Check sheet for the drawn part. Datum: minimum x, y, z corner. Units: mm. Round coordinates to 2 decimals unless told otherwise and drop trailing zeros. Loops run counter-clockwise (first coordinate to the right, second up) from the corner with the lowest first, then second, coordinate; pieces in that order, holes last. Notation, with made-up numbers: (-13.5, 25) -> (35.5, 25) arc R22 ccw to (35.5, 46) -> close; hole circle Ø7 at (-3.75, 18). An arc over 180 degrees is marked (long way). Write item = value, one per line. Start each with the question number.
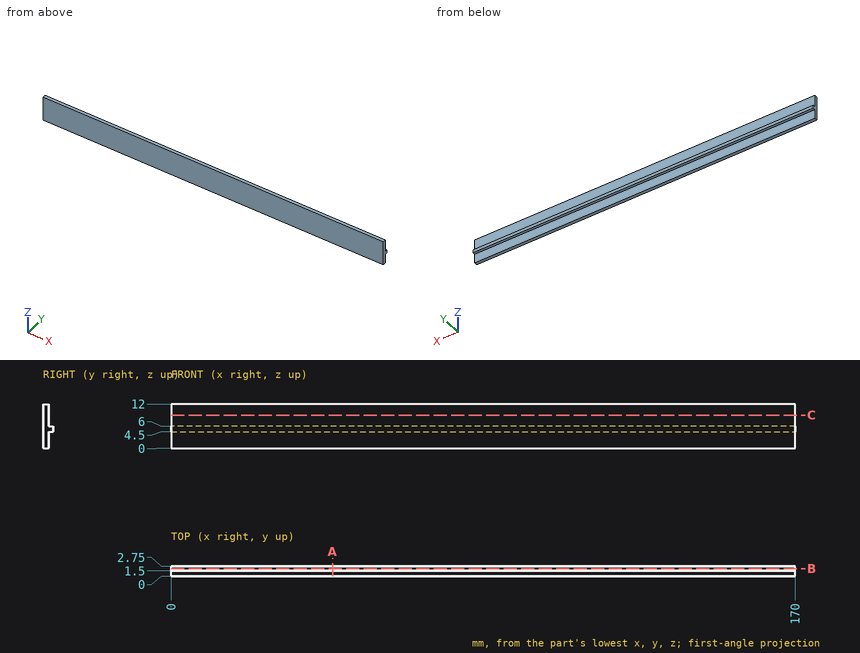
(1) Scan lines: line 1 (Y direction, x = 39.5, z = 7.5); line 2 (Z direction, x = 31, y = 2.6). Record each from-to range of solid material in increasing order. Write a range as [from, to].
(2) Section check A-A on x = 44. Enter the section's corners in (y, z).
(3) Depth check by flat-ended pin: pin 1 Ø1 at (x, z) = (44, 3) entering from +Y. Enter the tip coordinate at first touch or a pass-through.
(4) Section check C-C on z = 9. Enter the section's corners in (x, y), then the cut area to 3 significant figures.
(5) Section check B-B on y = 2.05. Enter the section's corners in (x, z).
Computed values:
q1.line_1 = [0, 1.5]
q1.line_2 = [4.5, 6]
q2.outline = (0, 0) -> (1.5, 0) -> (1.5, 4.5) -> (2.75, 4.5) -> (2.75, 6) -> (1.5, 6) -> (1.5, 12) -> (0, 12) -> close
q3.pin_1 = 1.5
q4.outline = (0, 0) -> (170, 0) -> (170, 1.5) -> (0, 1.5) -> close
q4.area = 255 mm²
q5.outline = (0, 4.5) -> (170, 4.5) -> (170, 6) -> (0, 6) -> close
